```python
from build123d import *

# Parameters (mm, degrees)
BOX001_W          = 71.8
BOX001_H          = 1
BOX001_DEPTH      = 9.5
CYLINDER004_R     = 7.9
CYLINDER004_DEPTH = 1.7
BOX_W             = 71.8
BOX_H             = 9.5
BOX_DEPTH         = 1


with BuildPart() as obj1:
    # Box001 → Box001 (new body)
    with BuildSketch(Plane(origin=(-40, 36.6, 10.375), x_dir=(1, 0, 0), z_dir=(0, 0, 1))):
        with Locations((35.9, 0.5)):
            Rectangle(BOX001_W, BOX001_H)
    extrude(amount=BOX001_DEPTH)


with BuildPart() as obj2:
    # Cylinder004 → Cylinder004 (new body)
    with BuildSketch(Plane(origin=(31.8, 36.6, 15.125), x_dir=(0, 0, -1), z_dir=(1, 0, 0))):
        Circle(CYLINDER004_R)
    extrude(amount=CYLINDER004_DEPTH)


with BuildPart() as fusion015:
    # Box → Box (new body)
    with BuildSketch(Plane(origin=(-40, 31.85, 14.625), x_dir=(1, 0, 0), z_dir=(0, 0, 1))):
        with Locations((35.9, 4.75)):
            Rectangle(BOX_W, BOX_H)
    extrude(amount=BOX_DEPTH)

    # Fusion015: union obj1, obj2
    add(obj1.part)
    add(obj2.part)


solid = fusion015.part
```
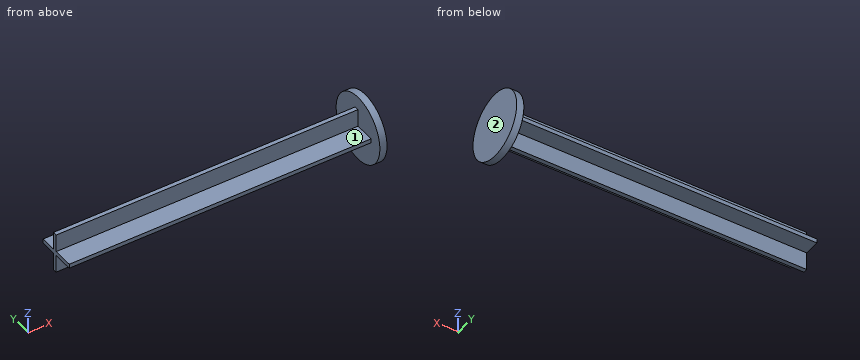
The listing builds one solid part. Answer for the finished solid, in the listing's coordinates (mm). Face numbers are marked on the shaded views. A direction names the side the tool comes from. Coordinates: 2 decimals unless noted, no trailing zeros. Write each loop counter-clockwise with the first axis right and the second up, starting at its lowest first coordinate (ties: lowest second). Pieces come first, ordered by that corner, then holes. Notation, with made-up numbers: (-27, 4) - (29, 4) arc R21 cw to (29, 18) - close; hole circle Ø9 at (6.5, 73.5). An arc over 180 degrees is marked (long way). Return JSON: item names as keys, results as strings. Group by question number.
Q1. The part is cut by section B-B on z = 14. Write down the section's boundary in (x, y).
Q2. The part is cut by section C-C on y = 34.25. Write down the section's boundary in (x, z) (3 decimals), and give its area (3 significant figures).
Q3. The part is cut by section A-A on x = 25. Write down the section's boundary in (y, z) (3 decimals).
Q4. Find the intervals of material crossed by line 1 along X through (y, z) = (33.75, 8); line 2 along Y through (x, z) = (-22, 19.75); line 3 along Z through (x, y) = (-11, 32.75) (3 decimals), in increasing order. Write a range as [from, to].
Q5. Which of the six approach directions +Z, -Z, +X, -X, +Y, -Y give full straight-line access (tool end or side, diameter ignored) to the marked faces 1 and 2?
Q6. Flat-ended cylindrical pins translate along their axes: pin 1 Ø2 at (x, y) = (7, 36) entering from -Z (3 decimals); pin 2 Ø3 at (x, y) = (7, 39.5) entering from +Z (3 decimals); pin 3 Ø1.3 at (x, z) = (-13, 17) entering from +Y. Find the tip coordinate at first contact, or state that the pin passes through.
Evaluation:
{
 "1": {"outline": "(-40, 36.6) - (31.8, 36.6) - (31.8, 28.78) - (33.5, 28.78) - (33.5, 44.42) - (31.8, 44.42) - (31.8, 37.6) - (-40, 37.6) - close"},
 "2": {"outline": "(-40, 14.625) - (31.8, 14.625) - (31.8, 7.583) - (33.5, 7.583) - (33.5, 22.667) - (31.8, 22.667) - (31.8, 15.625) - (-40, 15.625) - close", "area": "97.4 mm2"},
 "3": {"outline": "(31.85, 14.625) - (36.6, 14.625) - (36.6, 10.375) - (37.6, 10.375) - (37.6, 14.625) - (41.35, 14.625) - (41.35, 15.625) - (37.6, 15.625) - (37.6, 19.875) - (36.6, 19.875) - (36.6, 15.625) - (31.85, 15.625) - close"},
 "4": {"line 1": "x = [31.8, 33.5]", "line 2": "y = [36.6, 37.6]", "line 3": "z = [14.625, 15.625]"},
 "5": {"face 1": "+Z, -X, -Y", "face 2": "+Z, -Z, +X, +Y, -Y"},
 "6": {"pin 1": "stops at z = 10.375", "pin 2": "stops at z = 15.625", "pin 3": "stops at y = 37.6"}
}
